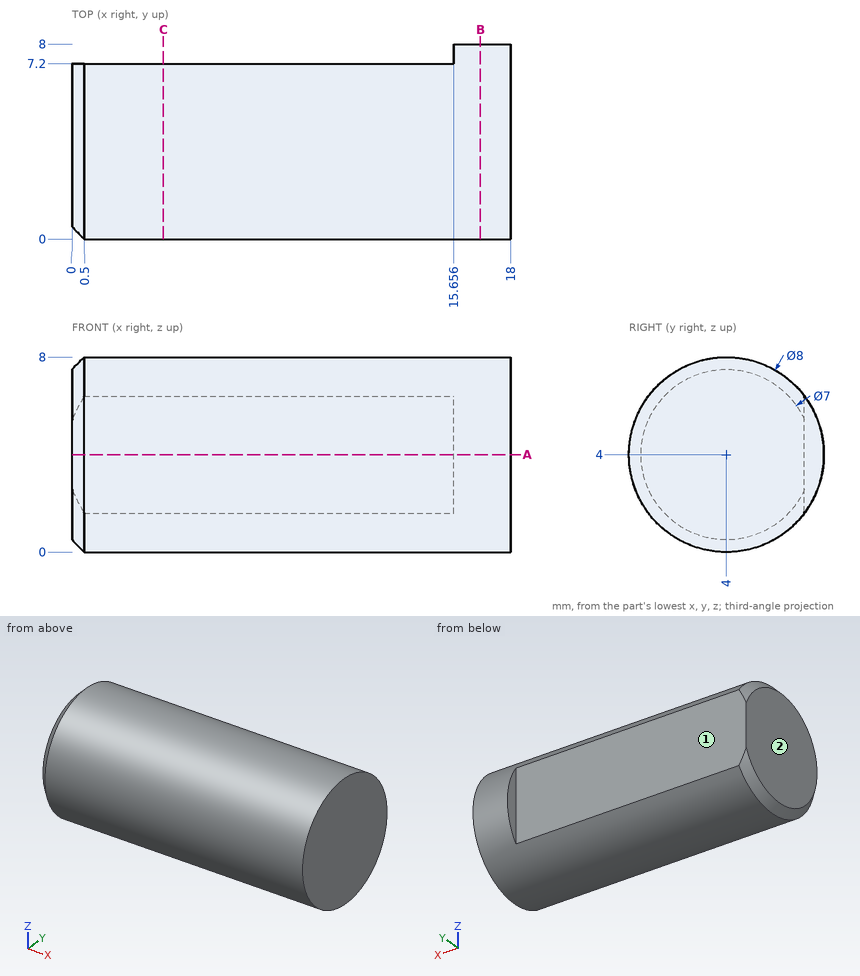
Study the drawing (mm; zero at the part's minimum x, y, z) and answer. A direction names the side the tool comes from. Round coordinates to 2 decimals unless told otherwise and drop trailing zeros. Order: outer loops, then holes, each group sorted by start corner. A loop starts at its lowest first (then second) coordinate and runs counter-clockwise, first axis right, second up. Notation, with made-up numbers: (68.25, -38.5) -> (91.25, -38.5) arc R22 cw to (91.25, -27.5) -> close; hole circle Ø9 at (16.5, 9.25). An arc over 180 degrees is marked (long way). Answer as CSV lines item,"result". Start each with the question number.
(1) A tool of negligible diameter and unlimited length cuts with its end or side. For the marked faces 1 and 2, from which of +Z, -Z, +X, -X, +Y, -Y can it reach the whole face along a straight path? Write none if from no direction.
(2) The part is cut by section C-C (x = 3.75). Determine the outline of the cut face in (y, z).
(3) Flat-ended cylindrical pins translate along their axes: pin 1 Ø4 at (x, y) = (10.5, 1.5) entering from -Z; pin 2 Ø1.5 at (x, z) = (4, 5) entering from +Y; pin 3 Ø1 at (x, y) = (5, 1.5) entering from -Z; pin 4 Ø3 at (y, z) = (3.5, 5.5) entering from -X. Find the tip coordinate at first contact, or state that the pin passes through.
(4) The part is cut by section A-A (z = 4). Determine the outline of the cut face in (x, y).
(5) The part is cut by section B-B (x = 16.75). Determine the outline of the cut face in (y, z), then the cut area to 3 significant figures.
(6) Find the intervals of material crossed by probe 1 along Z at (x, y) = (4, 6.25); probe 2 along Y at (x, z) = (1, 3.25); probe 3 along Z at (x, y) = (12.5, 2.75), in increasing order. Write a range as from..to.
Evaluation:
1,face 1,"+Z, -Z, -X, +Y"
1,face 2,"+Z, -Z, -X, +Y, -Y"
2,outline,"(7.2, 1.6) -> (7.2, 6.4) arc R4 ccw (long way) to start"
3,pin 1,"z = 0.03"
3,pin 2,"y = 7.2"
3,pin 3,"z = 0.54"
3,pin 4,"x = 0"
4,outline,"(0, 0.5) -> (0.5, 0) -> (18, 0) -> (18, 8) -> (15.66, 8) -> (15.66, 7.2) -> (0, 7.2) -> close"
5,outline,"circle Ø8 at (4, 4)"
5,area,"50.3 mm²"
6,probe 1,"0.69..7.31"
6,probe 2,"0.07..7.2"
6,probe 3,"0.2..7.8"
